Here's the drawing with two shaded views (mm, measured from the low corner). I have some questions. A direction names the side the tool comes from. Coordinates: 2 decimals unless noted, no trailing zeros. Write each loop counter-clockwise with the first axis right and the second up, starting at its lowest first coordinate (ties: lowest second). Pieces come first, ordered by that corner, then holes. Notation, with made-up numbers: (51.25, 75.25) -> (106.25, 75.25) arc R13 cw to (106.25, 79.25) -> close; hole circle Ø10 at (59.25, 29.5). An arc over 180 degrees is marked (long way). Put each result on its own line as item: value. Start each with the question number.
Item 1: On a 3-axis mill with a long thin cutter (end or side, diameter ignored), from which of +Z, -Z, +X, -X, +Y, -Y can I reach the whole of each face in a straight line? I mean the marked faces 1, 2 and 3. Say none if no direction works.
Item 2: I want a section at A-A, the plane z = 2.5. List the corners of the cut face in (x, y) for me, then the cut area to 3 significant figures.
Item 3: For pin 1 (3.5 mm diameter, centred on x = 15.5, z = 2, fed in from -Y); pin 2 (2.5 mm diameter, centred on x = 11.5, z = 1, fed in from +Y); pin 3 (1.5 mm diameter, centred on y = 19, z = 4.5, fed in from +X), each with a flat end and sliding along its axis, tell me the tip position at first contact or that it passes through.
Item 4: I need wall thicknesses on line 1 (Y direction, x = 13.5, z = 1.6); line 2 (Y direction, x = 13.5, z = 3.05); line 3 (Z direction, x = 25.75, y = 8.5). Which ranges of each line are inside material? Lowest first, please. Write a range as [from, to].
Item 5: I want a section at D-D, the plane z = 5. List the corners of the cut face in (x, y) for me (1 decimal).
Item 6: I want a section at C-C, the plane y = 4.75. List the corners of the cut face in (x, z) for me (1 decimal).
Item 7: I want a section at B-B, the plane x = 13.5. List the corners of the cut face in (y, z) for me, then the cut area to 3 significant figures.
Item 8: If we mould it in two halves opening along X, with no side actions, what happens to the marked faces 4, 5 and 6? For each: released by +X, released by -X, zero draft, split by the parting line, or undercut.
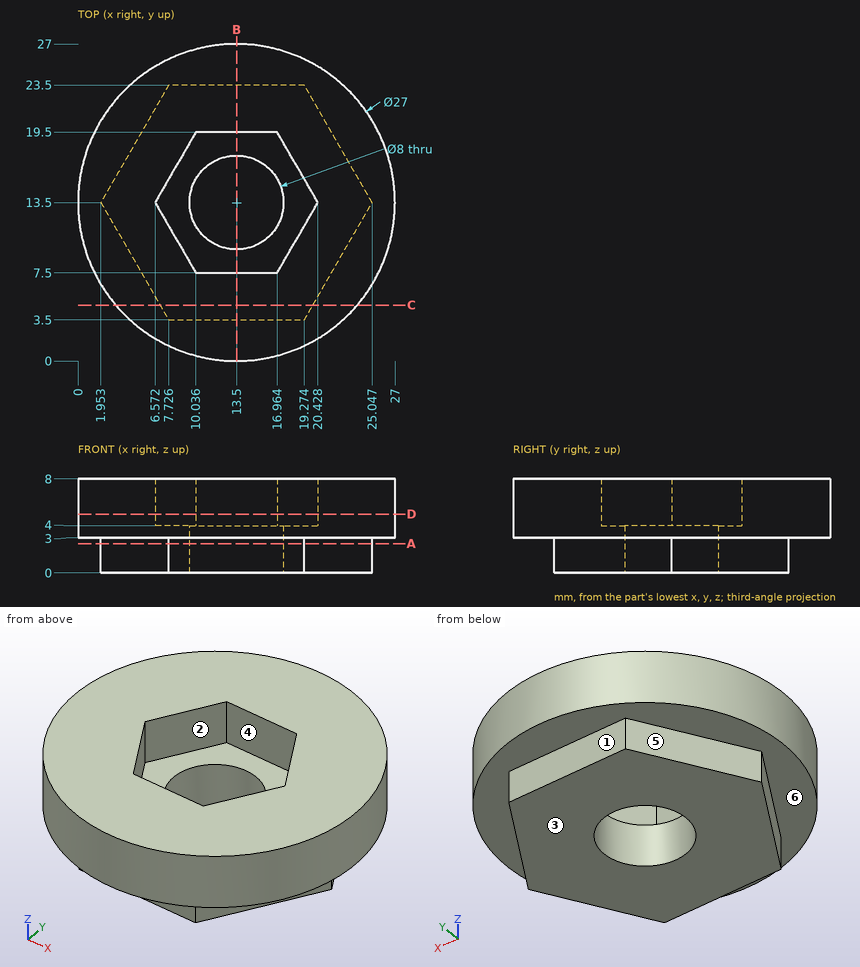
Calculated:
1. face 1: -Z, +X, -X, +Y
1. face 2: +Z
1. face 3: -Z, +X, -X, +Y, -Y
2. outline: (1.95, 13.5) -> (7.73, 3.5) -> (19.27, 3.5) -> (25.05, 13.5) -> (19.27, 23.5) -> (7.73, 23.5) -> close; hole circle Ø8 at (13.5, 13.5)
2. area: 296 mm2
3. pin 1: stops at y = 0.01
3. pin 2: stops at y = 23.5
3. pin 3: stops at x = 26.14
4. line 1: y = [3.5, 9.5], [17.5, 23.5]
4. line 2: y = [0, 9.5], [17.5, 27]
4. line 3: z = [3, 8]
5. outline: circle Ø27 at (13.5, 13.5); hole (6.6, 13.5) -> (10, 7.5) -> (17, 7.5) -> (20.4, 13.5) -> (17, 19.5) -> (10, 19.5) -> close
6. outline: (3.2, 3) -> (7, 3) -> (7, 0) -> (20, 0) -> (20, 3) -> (23.8, 3) -> (23.8, 8) -> (3.2, 8) -> close
7. outline: (0, 3) -> (3.5, 3) -> (3.5, 0) -> (9.5, 0) -> (9.5, 4) -> (7.5, 4) -> (7.5, 8) -> (0, 8) -> close; (17.5, 0) -> (23.5, 0) -> (23.5, 3) -> (27, 3) -> (27, 8) -> (19.5, 8) -> (19.5, 4) -> (17.5, 4) -> close
7. area: 115 mm2
8. face 4: undercut
8. face 5: released by -X
8. face 6: zero draft
